Solid Edge part; units mm, degrees
sketch "Sketch1" plane through (0, 0, 0) normal (0, -1, 0) x (1, 0, 0)
  line L0 (-62.8578, 12.4874) -> (87.1422, 12.4874)
  line L1 (87.1422, 12.4874) -> (-62.8578, 162.4874)
  line L2 (-62.8578, 162.4874) -> (-62.8578, 12.4874)
  dimension "D1" = 62.8578
  dimension "D2" = 62.8578
extrude "Protrusion1" add sketch "Sketch1" against normal blind 10
sketch "Sketch2" plane through (12.1422, 10, 87.4874) normal (0, 1, 0) x (-1, 0, 0)
  circle A0 centre (70, 25) radius 2.6
  circle A1 centre (70, -15) radius 2.6
  circle A2 centre (70, -55) radius 2.6
  circle A3 centre (70, 55) radius 2.6
  dimension "D1" = 70
extrude "Cutout1" cut sketch "Sketch2" against normal through all
mirror "Mirror1" about plane through (-9.8248, 5, 65.5204) normal (-0.7071, 0, 0.7071) of "Cutout1"
Source: CAD feature listing. Evaluate the final solid. Frame: model axes, mm. Round coordinates to 2 decimals unless told otherwise and drop trailing zeros. Loops run counter-clockwise (first coordinate to the right, second up) from the corner with the lowest first, then second, coordinate; pieces in that order, holes last. Notation, with made-up numbers: M 24,11.25 L 67,11.25 A13 cw 67,29.25 Z; hole C -18.75,82 d2. An arc over 180 degrees is marked long. Use a Markdown table: item, result. Add a question column.
1. Contact query for flat-ended pins moving along their axis: P1, Ø5, axis at y = 8, z = 75.5, coming from the +X side; P2, Ø6, axis at y = 8.5, z = 38.5, coming from the +X side; P3, Ø6, axis at y = 2.5, z = 108.5, coming from the +X side. Output: stop coordinate, or through.
2. Line query: line 1 (X direction, y = 3.5, z = 34.5); line 2 (Z direction, x = -0.5, y = 9.5); line 3 (Z direction, x = 37.5, y = 8.75). Output: solid intervals per line, ascending.
3. Section query A-A on y = 1.5. Give the number of separate pieces and of enclosed holes in the cut face, then the cut area to 3 significant figures.
4. Section query B-B on x = -9. Return the cut outline in (y, z), then the cut area to 3 significant figures.
5. Section query C-C on z = 105.5. Return the cut outline in (x, y).
Reported:
| question | item | result |
|---|---|---|
| 1 | P1 | stops at x = 26.63 |
| 1 | P2 | stops at x = 64.13 |
| 1 | P3 | stops at x = -5.87 |
| 2 | line 1 | x = -62.86 to -59.5, -56.21 to 65.13 |
| 2 | line 2 | z = 12.49 to 16.39, 18.58 to 100.13 |
| 2 | line 3 | z = 12.49 to 14.91, 20.06 to 62.13 |
| 3 | separate pieces | 1 |
| 3 | enclosed holes | 8 |
| 3 | area | 11,100 mm² |
| 4 | outline | M 0,12.49 L 10,12.49 L 10,108.63 L 0,108.63 Z |
| 4 | area | 961 mm² |
| 5 | outline | M -62.86,0 L -5.87,0 L -5.87,10 L -62.86,10 Z |
